```python
from build123d import *

# Parameters (mm, degrees)
ESBO_O1_W             = 20
ESBO_O1_H             = 20
ESBO_O1_W_2           = 16
ESBO_O1_H_2           = 16
EXTRUS_O_FINA1_DEPTH  = 310
ESBO_O4_R             = 2.85
ESBO_O4_R_2           = 1.6
CORTE_EXTRUS_O2_DEPTH = 21
ESBO_O5_R             = 2.6
CORTE_EXTRUS_O5_DEPTH = 21
ESBO_O6_R             = 2.1
CORTE_EXTRUS_O6_DEPTH = 21


with BuildPart() as part:
    # Esboço1 → Extrusão-Fina1 (new body)
    with BuildSketch(Plane(origin=(0, 0, 0), x_dir=(1, 0, 0), z_dir=(0, 1, 0))):
        with Locations((10, 10)):
            Rectangle(ESBO_O1_W, ESBO_O1_H)
        with Locations((10, 10)):
            Rectangle(ESBO_O1_W_2, ESBO_O1_H_2, mode=Mode.SUBTRACT)
    extrude(amount=EXTRUS_O_FINA1_DEPTH)

    # Esboço4 → Corte-extrusão2 (cut, through all)
    with BuildSketch(Plane.XY):
        with Locations((10, 299)):
            Circle(ESBO_O4_R)
        with Locations((10, 291)):
            Circle(ESBO_O4_R_2)
        with Locations((10, 307)):
            Circle(ESBO_O4_R_2)
    extrude(amount=-CORTE_EXTRUS_O2_DEPTH, mode=Mode.SUBTRACT)

    # Esboço5 → Corte-extrusão5 (cut, through all)
    with BuildSketch(Plane(origin=(0, 0, -20), x_dir=(-1, 0, 0), z_dir=(0, 0, -1))):
        with Locations((-10, 5)):
            Circle(ESBO_O5_R)
        with Locations((-10, 27)):
            Circle(ESBO_O5_R)
    extrude(amount=-CORTE_EXTRUS_O5_DEPTH, mode=Mode.SUBTRACT)

    # Esboço6 → Corte-extrusão6 (cut, through all)
    with BuildSketch(Plane.ZY):
        with Locations((-10, 16)):
            Circle(ESBO_O6_R)
    extrude(amount=-CORTE_EXTRUS_O6_DEPTH, mode=Mode.SUBTRACT)


solid = part.part
```
Part model, mm, in its own coordinate system. A direction names the side the tool comes from. Give positions to 0.01 mm unless a question says otherwise; leave off trailing zeros. Order: outer loops, then holes, each group sorted by start corner. A loop starts at its lowest first (then second) coordinate and runs counter-clockwise, first axis right, second up. Notation, with made-up numbers: (20, 19.25) - (69, 19.25) arc R21 cw to (69, 58.25) - close; hole circle Ø9 at (46, 78). An arc over 180 degrees is marked (long way). Use one line per item in the form item = value.
Item 1: Slice it at A-A on x = 4.5. Give the cut face in (y, z).
Solution:
outline = (0, -20) - (310, -20) - (310, -18) - (0, -18) - close; (0, -2) - (310, -2) - (310, 0) - (0, 0) - close
Item 2: Slice it at C-C on y = 159. Give the cut face in (x, z), and give its area (3 significant figures).
Solution:
outline = (0, -20) - (20, -20) - (20, 0) - (0, 0) - close; hole (2, -18) - (18, -18) - (18, -2) - (2, -2) - close
area = 144 mm2
Item 3: Two-plate mould, pull along Z, no slides. Class faces 1 (the face through (10, 153, 0)), 2 (the face through (10, 153, -20)), 3 (the face through (7.52, 5.78, -1.01)), 4 (the face through (10, 153, -2)): released by +Z, released by -Z, zero draft, split by the parting line, or undercut.
Solution:
face_1 = released by +Z
face_2 = released by -Z
face_3 = zero draft
face_4 = undercut
Item 4: Slice it at B-B on y = 27. Give the cut face in (x, z), and give its area (3 significant figures).
Solution:
outline = (0, -20) - (7.4, -20) - (7.4, -18) - (2, -18) - (2, -2) - (7.4, -2) - (7.4, 0) - (0, 0) - close; (12.6, -20) - (20, -20) - (20, 0) - (12.6, 0) - (12.6, -2) - (18, -2) - (18, -18) - (12.6, -18) - close
area = 123 mm2
Item 5: Probe probe 1 along Y at (x, z) = (10, -1.4); probe 2 along X at (y, z) = (243.5, -17.5); probe 3 along Z at (x, y) = (4.75, 171). List the from-to ranges inside material, lowest first. Write a range as from..to.
Solution:
probe_1 = 0..2.4, 7.6..24.4, 29.6..289.4, 292.6..296.15, 301.85..305.4, 308.6..310
probe_2 = 0..2, 18..20
probe_3 = -20..-18, -2..0
Item 6: Which spindle directions (+Z, -Z, +X, -X, +Y, -Y) get a long thin tool onto all of the face, cutting with end or side? Do faces 5 (the face through (2, 153, -10)), 6 (the face through (0, 153, -10)). Say none if no direction does.
Solution:
face_5 = +Y, -Y
face_6 = +Z, -Z, -X, +Y, -Y
Item 7: Slice it at D-D on y = 299. Give the cut face in (x, z).
Solution:
outline = (0, -20) - (7.15, -20) - (7.15, -18) - (2, -18) - (2, -2) - (7.15, -2) - (7.15, 0) - (0, 0) - close; (12.85, -20) - (20, -20) - (20, 0) - (12.85, 0) - (12.85, -2) - (18, -2) - (18, -18) - (12.85, -18) - close
